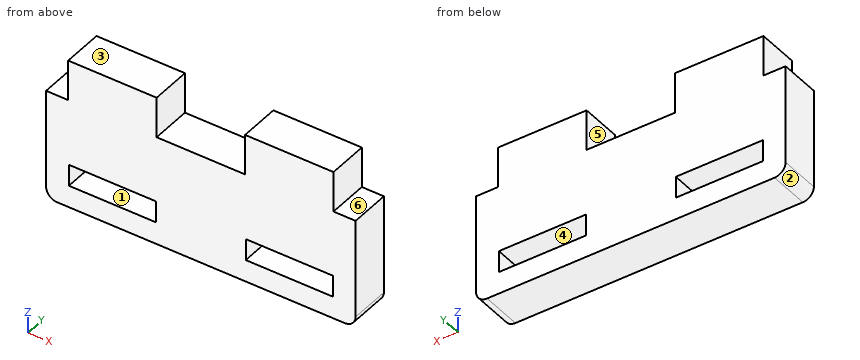
```python
from build123d import *

# Parameters (mm, degrees)
SKETCH1_W           = 12.5
SKETCH1_H           = 3.0988
BOSS_EXTRUDE1_DEPTH = 5.842
FILLET1_R           = 1.5875


with BuildPart() as part:
    # Sketch1 → Boss-Extrude1 (new body)
    with BuildSketch(Plane(origin=(0, 0, 0), x_dir=(1, 0, 0), z_dir=(0, 1, 0))):
        Polygon((22.225, -4.7625), (19.05, -4.7625), (19.05, -10.6045), (6.35, -10.6045), (6.35, -4.7625), (-6.35, -4.7625), (-6.35, -10.6045), (-19.05, -10.6045), (-19.05, -4.7625), (-22.225, -4.7625), (-22.225, 4.7625), (-22.225, 7.8613), (-22.225, 11.0363), (22.225, 11.0363), (22.225, 7.8613), (22.225, 4.7625), align=None)
        with Locations((12.7, 6.3119)):
            Rectangle(SKETCH1_W, SKETCH1_H, mode=Mode.SUBTRACT)
        with Locations((-12.7, 6.3119)):
            Rectangle(SKETCH1_W, SKETCH1_H, mode=Mode.SUBTRACT)
    extrude(amount=BOSS_EXTRUDE1_DEPTH)

    # Fillet1
    fillet1_edges = [part.edges().sort_by_distance(p)[0] for p in [
        (-22.225, 2.921, -11.0363),
        (22.225, 2.921, -11.0363),
    ]]
    fillet(fillet1_edges, radius=FILLET1_R)


solid = part.part
```
Could you check a few things on this model? Use its own coordinates, in mm. Face numbers are marked on the shaded views. A direction names the side the tool comes from. Coordinates: 2 decimals unless noted, no trailing zeros. Loops run counter-clockwise (first coordinate to the right, second up) from the corner with the lowest first, then second, coordinate; pieces in that order, holes last. Notation, with made-up numbers: M 81,55 L 90,55 A14 cw 90,60 Z; hole C 6,57 d8. An arc over 180 degrees is marked long. Put each result on its own line as item: value. Start each with the question number.
(1) For the marked faces 4, 5 and 6, which set-ups out of +Z, -Z, +X, -X, +Y, -Y let a thin tool reach every point of the face, with its end or its side?
(2) Will this pin go through, and if not, where does the flat tip stop? P1, Ø3, axis at x = 3, y = 3.5, coming from the +Z side.
(3) I need wall thicknesses on line 1 (X direction, y = 2.1, z = -6) (3 decimals); line 2 (X direction, y = 1.9, z = 8); line 3 (Z direction, x = -9, y = 2.3). Which ranges of each line are inside material? Lowest first, please. Write a range as from..to.
(4) Suppose I cut it at B-B on x = -11.5. Please give me the cut outline in (y, z), then the cut area to 3 significant figures.
(5) Suppose I cut it at C-C on x = -3. Please give me the cut outline in (y, z), then the cut area to 3 significant figures.
(6) Thinking about a two-plate mould opening in Z: for the marked faces 1, 2 and 3, which applies, pulls with the +Z half, pulls with the -Z half, needs draft (parallel to the pull), parting line crosses it, or undercut?
(7) Suppose I cut it at A-A on y = 4.5. Count the separate pieces of the cut face and the enclosed holes in it, then the cut area to 3 significant figures.
Solutions:
1. face 4: +Y, -Y
1. face 5: +Z, +Y, -Y
1. face 6: +Z, +X, +Y, -Y
2. P1: stops at z = 4.76
3. line 1: x = -22.225..-18.95, -6.45..6.45, 18.95..22.225
3. line 2: x = -19.05..-6.35, 6.35..19.05
3. line 3: z = -11.04..-7.86, -4.76..10.6
4. outline: M 0,-11.04 L 5.84,-11.04 L 5.84,-7.86 L 0,-7.86 Z; M 0,-4.76 L 5.84,-4.76 L 5.84,10.6 L 0,10.6 Z
4. area: 108 mm2
5. outline: M 0,-11.04 L 5.84,-11.04 L 5.84,4.76 L 0,4.76 Z
5. area: 92.3 mm2
6. face 1: undercut
6. face 2: pulls with the -Z half
6. face 3: pulls with the +Z half
7. separate pieces: 1
7. enclosed holes: 2
7. area: 772 mm2
